```python
from build123d import *

# Parameters (mm, degrees)
SKETCH1_W           = 130
SKETCH1_H           = 227
SKETCH1_W_2         = 87
SKETCH1_H_2         = 25
BOSS_EXTRUDE1_DEPTH = 3
SKETCH2_W           = 10
SKETCH2_H           = 3
BOSS_EXTRUDE2_DEPTH = 3
LPATTERN1_COUNT     = 6
LPATTERN1_PITCH     = 20
SKETCH3_W           = 10
SKETCH3_H           = 3
BOSS_EXTRUDE3_DEPTH = 3
LPATTERN2_COUNT     = 6
LPATTERN2_PITCH     = 20
SKETCH4_W           = 3
SKETCH4_H           = 10
BOSS_EXTRUDE4_DEPTH = 3
LPATTERN3_COUNT     = 11
LPATTERN3_PITCH     = 20
SKETCH5_W           = 3
SKETCH5_H           = 10
BOSS_EXTRUDE5_DEPTH = 3
LPATTERN4_COUNT     = 11
LPATTERN4_PITCH     = 20
SKETCH6_W           = 3
SKETCH6_H           = 10
CUT_EXTRUDE1_DEPTH  = 3
LPATTERN5_COUNT     = 11
LPATTERN5_PITCH     = 20


with BuildPart() as part:
    # Sketch1 → Boss-Extrude1 (new body)
    with BuildSketch(Plane.XY):
        with Locations((65, 113.5)):
            Rectangle(SKETCH1_W, SKETCH1_H)
        with Locations((78.5, 20.5)):
            Rectangle(SKETCH1_W_2, SKETCH1_H_2, mode=Mode.SUBTRACT)
        with Locations((78.5, 206.5)):
            Rectangle(SKETCH1_W_2, SKETCH1_H_2, mode=Mode.SUBTRACT)
    extrude(amount=BOSS_EXTRUDE1_DEPTH)

    # Sketch2 → Boss-Extrude2 (add)
    with BuildSketch(Plane.XZ):
        with Locations((15, 1.5)):
            Rectangle(SKETCH2_W, SKETCH2_H)
    boss_extrude2 = extrude(amount=BOSS_EXTRUDE2_DEPTH)

    # LPattern1: Boss-Extrude2 ×6
    with Locations(*[(i * LPATTERN1_PITCH, 0, 0) for i in range(1, LPATTERN1_COUNT)]):
        add(boss_extrude2)

    # Sketch3 → Boss-Extrude3 (add)
    with BuildSketch(Plane(origin=(0, 227, 0), x_dir=(1, 0, 0), z_dir=(0, 1, 0))):
        with Locations((15, -1.5)):
            Rectangle(SKETCH3_W, SKETCH3_H)
    boss_extrude3 = extrude(amount=BOSS_EXTRUDE3_DEPTH)

    # LPattern2: Boss-Extrude3 ×6
    with Locations(*[(i * LPATTERN2_PITCH, 0, 0) for i in range(1, LPATTERN2_COUNT)]):
        add(boss_extrude3)

    # Sketch4 → Boss-Extrude4 (add)
    with BuildSketch(Plane(origin=(130, 0, 0), x_dir=(0, 0, -1), z_dir=(1, 0, 0))):
        with Locations((-1.5, 15)):
            Rectangle(SKETCH4_W, SKETCH4_H)
    boss_extrude4 = extrude(amount=BOSS_EXTRUDE4_DEPTH)

    # LPattern3: Boss-Extrude4 ×11
    with Locations(*[(0, i * LPATTERN3_PITCH, 0) for i in range(1, LPATTERN3_COUNT)]):
        add(boss_extrude4)

    # Sketch5 → Boss-Extrude5 (add)
    with BuildSketch(Plane.ZY):
        with Locations((1.5, 15)):
            Rectangle(SKETCH5_W, SKETCH5_H)
    boss_extrude5 = extrude(amount=BOSS_EXTRUDE5_DEPTH)

    # LPattern4: Boss-Extrude5 ×11
    with Locations(*[(0, i * LPATTERN4_PITCH, 0) for i in range(1, LPATTERN4_COUNT)]):
        add(boss_extrude5)

    # Sketch6 → Cut-Extrude1 (cut)
    with BuildSketch(Plane.XY.offset(3)):
        with Locations((26.5, 15)):
            Rectangle(SKETCH6_W, SKETCH6_H)
    cut_extrude1 = extrude(amount=-CUT_EXTRUDE1_DEPTH, mode=Mode.SUBTRACT)

    # LPattern5: Cut-Extrude1 ×11
    with Locations(*[(0, i * LPATTERN5_PITCH, 0) for i in range(1, LPATTERN5_COUNT)]):
        add(cut_extrude1, mode=Mode.SUBTRACT)


solid = part.part
```
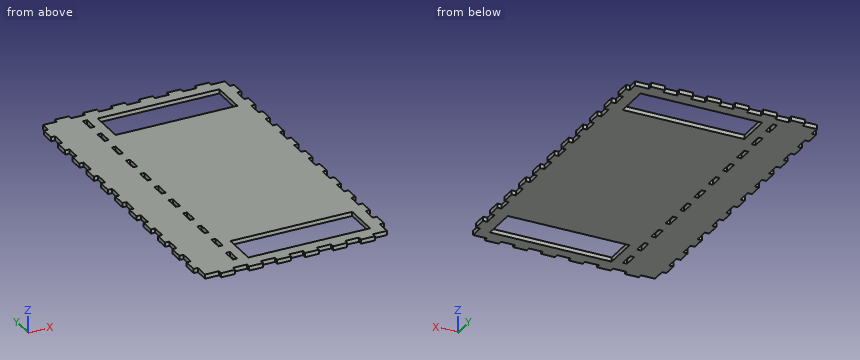
For this review, take the finished solid that the model builds, in its own axes (mm). Give positions to 0.01 mm unless a question says otherwise; leave off trailing zeros. Write each loop counter-clockwise with the first axis right and the second up, starting at its lowest first coordinate (ties: lowest second). Pieces come first, ordered by that corner, then holes.
Item 1: Wall thickness on probe 1 along Y at (x, z) = (77, 1.7); probe 2 along X at (y, z) = (19, 2.75); probe 3 along Y at (x, z) = (100.5, 1.8): over which ranges is each line inside the solid? List them lowest first.
Item 2: Take a section at A-A (x = 76). Give the boundary of the cut face in (y, z).
Item 3: Take a section at C-C (y = 153). Give the boundary of the cut face in (x, z).
Item 4: Take a section at B-B (y = 13.5). Give the boundary of the cut face in (x, z).
Item 5: Insertion check: P1, Ø0.9, axis at x = -1, z = 1.5, coming from the -Y side; P2, Ø10, axis at x = 118.5, y = 203, coming from the +Z side; P3, Ø1.5, axis at x = 4, z = 1, coming from the -Y side; P4, Ø0.9, axis at x = -1.5, z = 2, coming from the +Y side. Each pin has a flat end and moves straight along its axis. Give the tip position at first contact, or say it passes through.
Item 6: Take a section at D-D (z = 1.75). Give the number of separate pieces and of enclosed holes in the cut face, and give its area (4 significant figures).
Established:
1. probe 1: y = -3 to 8, 33 to 194, 219 to 230
1. probe 2: x = -3 to 25, 28 to 35, 122 to 133
1. probe 3: y = 0 to 8, 33 to 194, 219 to 227
2. outline: (-3, 0) - (8, 0) - (8, 3) - (-3, 3) - close; (33, 0) - (194, 0) - (194, 3) - (33, 3) - close; (219, 0) - (230, 0) - (230, 3) - (219, 3) - close
3. outline: (-3, 0) - (25, 0) - (25, 3) - (-3, 3) - close; (28, 0) - (133, 0) - (133, 3) - (28, 3) - close
4. outline: (-3, 0) - (25, 0) - (25, 3) - (-3, 3) - close; (28, 0) - (35, 0) - (35, 3) - (28, 3) - close; (122, 0) - (133, 0) - (133, 3) - (122, 3) - close
5. P1: stops at y = 10
5. P2: stops at z = 3
5. P3: stops at y = 0
5. P4: stops at y = 220
6. separate pieces: 1
6. enclosed holes: 13
6. area: 25,850 mm2
